from build123d import *

# Parameters (mm, degrees)
SKETCH1_W           = 38.1
SKETCH1_H           = 38.1
BOSS_EXTRUDE1_DEPTH = 12.7
FILLET1_R           = 2.54
SHELL1_T            = -3.175
FILLET2_R           = 2.54
BOSS_EXTRUDE2_DEPTH = 19.05


with BuildPart() as part:
    # Sketch1 → Boss-Extrude1 (new body)
    with BuildSketch(Plane(origin=(0, 0, 0), x_dir=(1, 0, 0), z_dir=(0, 1, 0))):
        Rectangle(SKETCH1_W, SKETCH1_H)
    extrude(amount=BOSS_EXTRUDE1_DEPTH)

    # Fillet1
    fillet1_edges = [part.edges().sort_by_distance(p)[0] for p in [
        (19.05, 6.35, 19.05),
        (-19.05, 6.35, 19.05),
        (-19.05, 6.35, -19.05),
        (19.05, 6.35, -19.05),
    ]]
    fillet(fillet1_edges, radius=FILLET1_R)

    # Shell1
    shell1_openings = [part.faces().sort_by_distance(p)[0] for p in [
        (0, 12.7, 0),
    ]]
    offset(amount=SHELL1_T, openings=shell1_openings, kind=Kind.INTERSECTION)

    # Fillet2
    fillet2_edges = [part.edges().sort_by_distance(p)[0] for p in [
        (15.875, 7.9375, -15.875),
        (-15.875, 7.9375, -15.875),
        (-15.875, 7.9375, 15.875),
        (15.875, 7.9375, 15.875),
    ]]
    fillet(fillet2_edges, radius=FILLET2_R)

    # Sketch2 → Boss-Extrude2 (add)
    with BuildSketch(Plane(origin=(0, 3.175, 0), x_dir=(1, 0, 0), z_dir=(0, 1, 0))):
        with BuildLine():
            Line((15.875, -13.335), (15.875, 13.335))
            ThreePointArc((15.875, 13.335), (15.131051224, 15.131051224), (13.335, 15.875))
            Line((13.335, 15.875), (-13.335, 15.875))
            ThreePointArc((-13.335, 15.875), (-15.131051224, 15.131051224), (-15.875, 13.335))
            Line((-15.875, 13.335), (-15.875, -13.335))
            ThreePointArc((-15.875, -13.335), (-15.131051224, -15.131051224), (-13.335, -15.875))
            Line((-13.335, -15.875), (13.335, -15.875))
            ThreePointArc((13.335, -15.875), (15.131051224, -15.131051224), (15.875, -13.335))
        make_face()
    extrude(amount=BOSS_EXTRUDE2_DEPTH)


solid = part.part
Design review of the part built by this model. Coordinates are the model's own, in mm. A direction names the side the tool comes from. Give positions to 0.01 mm unless a question says otherwise; leave off trailing zeros. Write each loop counter-clockwise with the first axis right and the second up, starting at its lowest first coordinate (ties: lowest second). Pieces come first, ordered by that corner, then holes. Notation, with made-up numbers: M 78,40.25 L 134,40.25 A15 cw 134,60.25 Z; hole C 58,-12 d6. An arc over 180 degrees is marked long. Answer as a JSON object with one key per item and string values. Group by question number.
1) We need section A-A (z = 4.5). Give the boundary of the cut face in (x, y) (3 decimals).
2) Tool access review of faces 4 (the face through (-15.875, 17, 0)), 5 (the face through (15.15, 17.4, -15.11)), 6 (the face through (15.11, 17.4, 15.15)): name each direction out of +Z, -Z, +X, -X, +Y, -Y from which nothing blocks a thin tool from reaching the whole face with its end or side.
3) Clearance check with flat-ended pins moving along their axes: pin 1 Ø3 at (x, y) = (-1, 18) entering from -Z (3 decimals); pin 2 Ø3 at (x, y) = (-5, 18.5) entering from +Z (3 decimals); pin 3 Ø10.5 at (y, z) = (19, -4) entering from -X (3 decimals). State where each tip first meets the part, or that it passes through.
4) We need section B-B (x = -5). Give the boundary of the cut face in (y, z) (3 decimals), and give its area (3 significant figures).
5) Mouldability with a two-part tool opening along X and no side actions: class faces 1 (the face through (0, 17, 15.875)), 2 (the face through (-18.326, 6.439, -18.286)), 3 (the face through (15.875, 17, 0)) as released by +X, released by -X, zero draft, split by the parting line, or undercut.
6) For line 1 along X through (y, z) = (18, -9) (3 decimals); line 2 along Y through (x, z) = (-10, 17.5), list the stretches that pass through material, from the lowest coordinate up.
Answer key:
{
 "1": {"outline": "M -19.05,0 L 19.05,0 L 19.05,12.7 L 15.875,12.7 L 15.875,22.225 L -15.875,22.225 L -15.875,12.7 L -19.05,12.7 Z"},
 "2": {"face 4": "+Z, -Z, -X, +Y", "face 5": "-Z, +X, +Y", "face 6": "+Z, +X, +Y"},
 "3": {"pin 1": "stops at z = -15.875", "pin 2": "stops at z = 15.875", "pin 3": "stops at x = -15.875"},
 "4": {"outline": "M 0,-19.05 L 12.7,-19.05 L 12.7,-15.875 L 22.225,-15.875 L 22.225,15.875 L 12.7,15.875 L 12.7,19.05 L 0,19.05 Z", "area": "786 mm²"},
 "5": {"face 1": "zero draft", "face 2": "released by -X", "face 3": "released by +X"},
 "6": {"line 1": "x = -15.875 to 15.875", "line 2": "y = 0 to 12.7"}
}
